Geometry check sheet. Reference: the model listing, model coordinates, mm. Face numbers are marked on the shaded views. Round coordinates to 2 decimals unless told otherwise and drop trailing zeros. Order: outer loops, then holes, each group sorted by start corner. A loop starts at its lowest first (then second) coordinate and runs counter-clockwise, first axis right, second up. Notation, with made-up numbers: (69, -3.5) - (124, -3.5) arc R26 ccw to (124, 32.5) - close; hole circle Ø8 at (-19, 7). An arc over 180 degrees is marked (long way). One line per question, with ' | ' between items. Start each with the question number.
Q1. Sectioned sample at A-A, the plane z = 0. Enter the section's corners in (x, y) (3 decimals).
Q2. Sectioned sample at B-B, the plane y = 7. Give the number of separate pieces and of enclosed holes in the cut face, then the cut area to 3 significant figures.
Q3. Mould release check, pull along X, two halves, no side actions. Record for the marked faces 1, 2 and 3: +X half, -X half, draft (parallel to the pull), parting line (faces both ways), or undercut.
Q4. Material ranges on line 1 along X through (y, z) = (12.75, 0) (3 decimals); line 2 along X through (y, z) = (18.25, 0); line 3 along Z through (x, y) = (40.5, 15), recorded low to high.
Q5. Sectioned sample at C-C, the plane x = 0. Enter the section's corners in (y, z).
Q6. Gauge pin test, flat ends, axial feed: P1, Ø3, axis at y = 4.5, z = 43, coming from the +X side; P2, Ø2, axis at y = 19.5, z = 79, coming from the -X side; P3, Ø3, axis at y = 16.5, z = 48, coming from the -X side. Record the tip position at first contact, or that the pin passes through.
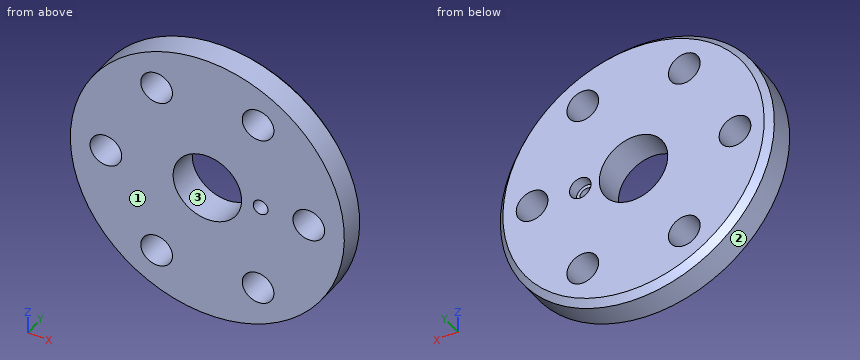
```python
from build123d import *

# Parameters (mm, degrees)
SKETCH1_R               = 108
SKETCH1_R_2             = 27
SKETCH1_R_3             = 12.5
BOSS_EXTRUDE1_DEPTH     = 25
CHAMFER1_SIZE           = 5
M12X0_35_TAPPED_HOLE2_D = 11.65
SKETCH4_R               = 8.5
CUT_EXTRUDE2_DEPTH      = 9


with BuildPart() as part:
    # Sketch1 → Boss-Extrude1 (new body)
    with BuildSketch(Plane(origin=(0, 0, 0), x_dir=(1, 0, 0), z_dir=(0, 1, 0))):
        with Locations(Location((0, 0, 0), (0, 0, 270))):
            Circle(SKETCH1_R)
        with Locations(Location((0, 0, 0), (0, 0, 270))):
            Circle(SKETCH1_R_2, mode=Mode.SUBTRACT)
        with Locations(Location((40, 69.282032303, 0), (0, 0, 270))):
            Circle(SKETCH1_R_3, mode=Mode.SUBTRACT)
        with Locations(Location((80, 0, 0), (0, 0, 270))):
            Circle(SKETCH1_R_3, mode=Mode.SUBTRACT)
        with Locations(Location((40, -69.282032303, 0), (0, 0, 270))):
            Circle(SKETCH1_R_3, mode=Mode.SUBTRACT)
        with Locations(Location((-40, -69.282032303, 0), (0, 0, 270))):
            Circle(SKETCH1_R_3, mode=Mode.SUBTRACT)
        with Locations(Location((-80, 0, 0), (0, 0, 270))):
            Circle(SKETCH1_R_3, mode=Mode.SUBTRACT)
        with Locations(Location((-40, 69.282032303, 0), (0, 0, 270))):
            Circle(SKETCH1_R_3, mode=Mode.SUBTRACT)
    extrude(amount=BOSS_EXTRUDE1_DEPTH)

    # Chamfer1
    chamfer1_edges = [part.edges().sort_by_distance(p)[0] for p in [
        (0, 25, -108),
    ]]
    chamfer(chamfer1_edges, length=CHAMFER1_SIZE)

    # M12x0.35 Tapped Hole2 (through all)
    with Locations(Plane(origin=(42, 0, 0), x_dir=(0, 0, -1), z_dir=(0, -1, 0))):
        with Locations((0, 0)):
            Hole(M12X0_35_TAPPED_HOLE2_D / 2)

    # Sketch4 → Cut-Extrude2 (cut)
    with BuildSketch(Plane(origin=(0, 25, 0), x_dir=(1, 0, 0), z_dir=(0, 1, 0))):
        with Locations(Location((42, 0, 0), (0, 0, 270))):
            Circle(SKETCH4_R)
    extrude(amount=-CUT_EXTRUDE2_DEPTH, mode=Mode.SUBTRACT)


solid = part.part
```
Determined:
1) outline: (-108, 0) - (-92.5, 0) - (-92.5, 25) - (-103, 25) - (-108, 20) - close; (-67.5, 0) - (-27, 0) - (-27, 25) - (-67.5, 25) - close; (27, 0) - (36.175, 0) - (36.175, 16) - (33.5, 16) - (33.5, 25) - (27, 25) - close; (47.825, 0) - (67.5, 0) - (67.5, 25) - (50.5, 25) - (50.5, 16) - (47.825, 16) - close; (92.5, 0) - (108, 0) - (108, 20) - (103, 25) - (92.5, 25) - close
2) separate pieces: 1 | enclosed holes: 8 | area: 31,300 mm2
3) face 1: draft | face 2: parting line | face 3: undercut
4) line 1: x = -108 to -92.5, -67.5 to -27, 27 to 36.175, 47.825 to 67.5, 92.5 to 108 | line 2: x = -108 to -92.5, -67.5 to -27, 27 to 33.5, 50.5 to 67.5, 92.5 to 108 | line 3: z = -100.12 to -81.77, -56.79 to -5.63, 5.63 to 56.79, 81.77 to 100.12
5) outline: (0, -108) - (20, -108) - (25, -103) - (25, -27) - (0, -27) - close; (0, 27) - (25, 27) - (25, 103) - (20, 108) - (0, 108) - close
6) P1: stops at x = 99.71 | P2: stops at x = -74.7 | P3: stops at x = -97.48
